Design review of the part shown in the three views and the two pictorial views. Dimensions are in mm from the part's minimum x, y and z. A direction names the side the tool comes from. Coordinates: 2 decimals unless noted, no trailing zeros. Write each loop counter-clockwise with the first axis right and the second up, starting at its lowest first coordinate (ties: lowest second). Pieces come first, ordered by that corner, then holes. Notation, with made-up numbers: (71.25, 57) - (101.25, 57) arc R29 ccw to (101.25, 82) - close; hole circle Ø7 at (79.5, 42). An arc over 180 degrees is marked (long way). Return JSON: item names as keys, results as strings. Group by question number.
(1) We need section D-D on x = 36.5. State the section outline as (y, z) points, then the cut area to 3 significant figures.
(2) We need section B-B on x = 9.8. State the section outline as (y, z) points.
(3) For pin 1 Ø1.2 at (x, z) = (41.5, 2.5) entering from +Y; pin 2 Ø1.5 at (x, z) = (33.5, 1.5) entering from +Y, all flat-tipped, find the tip position at first contact; note any pin that passes through.
(4) Draft analysis for pull direction X (two halves, no side actions). For the marked faces 1, 2 and 3, state which applies: released by +X, released by -X, zero draft, split by the parting line, or undercut.
(5) Tool access review of the marked faces 4, 5, 6, 7 and 8: name each direction out of +Z, -Z, +X, -X, +Y, -Y from which nothing blocks a thin tool from reaching the whole face with its end or side.
(6) We need section A-A on y = 28.1. State the section outline as (x, z) points, then the cut area to 3 significant figures.
(7) We need section C-C on z = 1.2. State the section outline as (x, y) points, then the cut area to 3 significant figures.
(8) To check wall thickness, follow L1, parallel to X at y = 27, z = 1.4; L2, parallel to X at y = 31, z = 1; L3, parallel to Y at x = 9.8, z = 1.4. State the ranges of each line that lie inside material, in increasing order. Write a range as from..to.
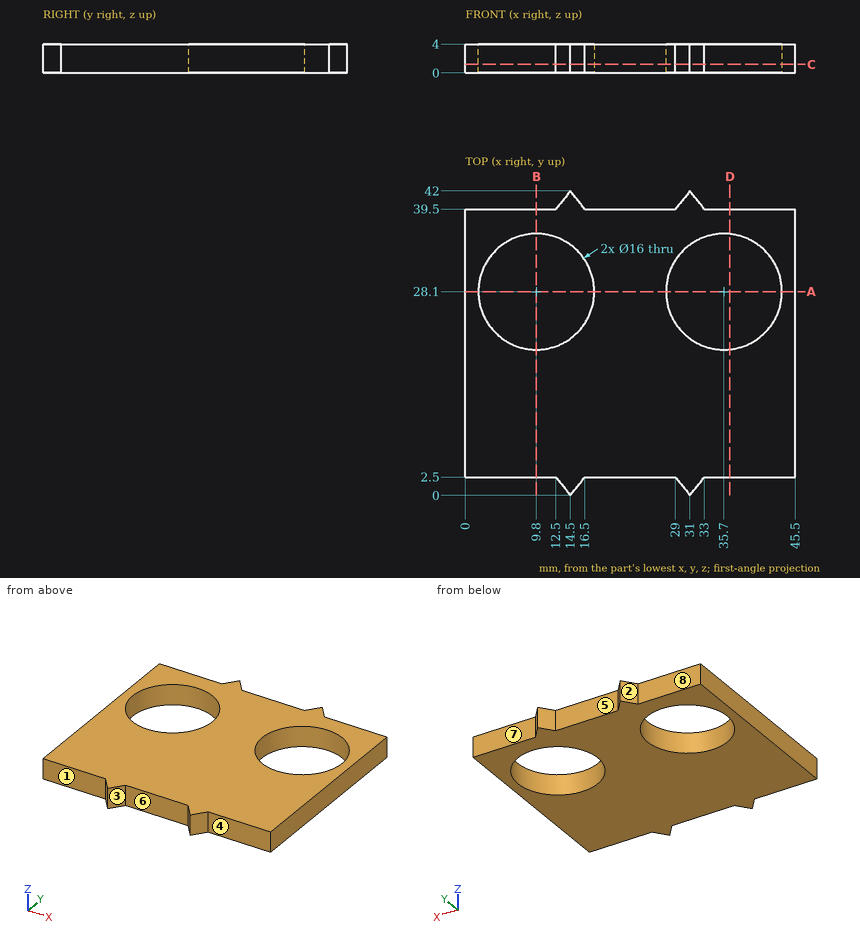
Ans:
{
 "1": {"outline": "(2.5, 0) - (20.14, 0) - (20.14, 4) - (2.5, 4) - close; (36.06, 0) - (39.5, 0) - (39.5, 4) - (36.06, 4) - close", "area": "84.3 mm²"},
 "2": {"outline": "(2.5, 0) - (20.1, 0) - (20.1, 4) - (2.5, 4) - close; (36.1, 0) - (39.5, 0) - (39.5, 4) - (36.1, 4) - close"},
 "3": {"pin 1": "y = 39.5", "pin 2": "y = 39.81"},
 "4": {"face 1": "zero draft", "face 2": "released by -X", "face 3": "undercut"},
 "5": {"face 4": "+Z, -Z, +X, -Y", "face 5": "+Z, -Z, +Y", "face 6": "+Z, -Z, -Y", "face 7": "+Z, -Z, +X, +Y", "face 8": "+Z, -Z, -X, +Y"},
 "6": {"outline": "(0, 0) - (1.8, 0) - (1.8, 4) - (0, 4) - close; (17.8, 0) - (27.7, 0) - (27.7, 4) - (17.8, 4) - close; (43.7, 0) - (45.5, 0) - (45.5, 4) - (43.7, 4) - close", "area": "54.0 mm²"},
 "7": {"outline": "(0, 2.5) - (12.5, 2.5) - (14.5, 0) - (16.5, 2.5) - (29, 2.5) - (31, 0) - (33, 2.5) - (45.5, 2.5) - (45.5, 39.5) - (33, 39.5) - (31, 42) - (29, 39.5) - (16.5, 39.5) - (14.5, 42) - (12.5, 39.5) - (0, 39.5) - close; hole circle Ø16 at (9.8, 28.1); hole circle Ø16 at (35.7, 28.1)", "area": "1,300 mm²"},
 "8": {"L1": "0..1.88, 17.72..27.78, 43.62..45.5", "L2": "0..2.34, 17.26..28.24, 43.16..45.5", "L3": "2.5..20.1, 36.1..39.5"}
}
